The model under review builds one solid part; all positions refer to its coordinate system, in mm. Face numbers are marked on the shaded views. Coordinates: 2 decimals unless noted, no trailing zeros.
1) For P1, Ø2, axis at y = 2, z = 29.5, coming from the -X side; P2, Ø2.5, axis at x = 5, z = 64, coming from the +Y side; P3, Ø2, axis at x = -2, z = 12, coming from the +Y side; P4, Ø6, axis at x = 6, z = 89, coming from the -Y side, all flat-tipped, find the tip position at first contact; note any pin that passes through.
2) Mouldability with a two-part tool opening along X and no side actions: class the marked faces 1, 2 and 3 as released by +X, released by -X, zero draft, split by the parting line, or undercut.
3) Add section A-A, the plane z = 40.5. Give the number of separate pieces and of enclosed holes in the cut face, then the cut area to 3 significant figures.
4) For line 1 (Y direction, x = 19, z = 88); line 2 (X direction, y = -21, z = 15); line 3 (X direction, y = -11.5, z = 65), list the stretches that pass through material, from the lowest coordinate up.
from build123d import *

# Parameters (mm, degrees)
EXTRUDE_1_DEPTH = 100


with BuildPart() as part:
    # 草图1 → 凸台-拉伸1 (new body)
    with BuildSketch(Plane.XY):
        with BuildLine():
            Line((23.205623676, 19.265775848), (23.205623676, 5.365775848))
            Line((23.205623676, 5.365775848), (22.405623676, 5.365775848))
            ThreePointArc((22.405623676, 5.365775848), (22.264202319, 5.307197204), (22.205623676, 5.165775848))
            Line((22.205623676, 5.165775848), (22.205623676, 4.365775848))
            Line((22.205623676, 4.365775848), (19.005623676, 4.365775848))
            ThreePointArc((19.005623676, 4.365775848), (18.793491641, 4.453643813), (18.705623676, 4.665775848))
            Line((18.705623676, 4.665775848), (18.705623676, 6.565775848))
            ThreePointArc((18.705623676, 6.565775848), (18.793491641, 6.777907882), (19.005623676, 6.865775848))
            Line((19.005623676, 6.865775848), (20.205623676, 6.865775848))
            ThreePointArc((20.205623676, 6.865775848), (20.912730457, 7.158669066), (21.205623676, 7.865775848))
            Line((21.205623676, 7.865775848), (21.205623676, 9.515775848))
            ThreePointArc((21.205623676, 9.515775848), (20.912730457, 10.222882629), (20.205623676, 10.515775848))
            Line((20.205623676, 10.515775848), (15.137604191, 10.515775848))
            Line((15.137604191, 10.515775848), (10.905623676, 6.283795332))
            Line((10.905623676, 6.283795332), (10.905623676, -7.752243637))
            Line((10.905623676, -7.752243637), (15.137604191, -11.984224152))
            Line((15.137604191, -11.984224152), (20.205623676, -11.984224152))
            ThreePointArc((20.205623676, -11.984224152), (20.912730457, -11.691330934), (21.205623676, -10.984224152))
            Line((21.205623676, -10.984224152), (21.205623676, -9.334224152))
            ThreePointArc((21.205623676, -9.334224152), (20.912730457, -8.627117371), (20.205623676, -8.334224152))
            Line((20.205623676, -8.334224152), (19.005623676, -8.334224152))
            ThreePointArc((19.005623676, -8.334224152), (18.793491641, -8.246356187), (18.705623676, -8.034224152))
            Line((18.705623676, -8.034224152), (18.705623676, -6.134224152))
            ThreePointArc((18.705623676, -6.134224152), (18.793491641, -5.922092118), (19.005623676, -5.834224152))
            Line((19.005623676, -5.834224152), (22.205623676, -5.834224152))
            Line((22.205623676, -5.834224152), (22.205623676, -6.634224152))
            ThreePointArc((22.205623676, -6.634224152), (22.264202319, -6.775645509), (22.405623676, -6.834224152))
            Line((22.405623676, -6.834224152), (23.205623676, -6.834224152))
            Line((23.205623676, -6.834224152), (23.205623676, -20.734224152))
            ThreePointArc((23.205623676, -20.734224152), (22.473390628, -22.501991105), (20.705623676, -23.234224152))
            Line((20.705623676, -23.234224152), (6.805623676, -23.234224152))
            Line((6.805623676, -23.234224152), (6.805623676, -22.434224152))
            ThreePointArc((6.805623676, -22.434224152), (6.747045032, -22.292802796), (6.605623676, -22.234224152))
            Line((6.605623676, -22.234224152), (5.805623676, -22.234224152))
            Line((5.805623676, -22.234224152), (5.805623676, -19.034224152))
            ThreePointArc((5.805623676, -19.034224152), (5.893491641, -18.822092118), (6.105623676, -18.734224152))
            Line((6.105623676, -18.734224152), (8.005623676, -18.734224152))
            ThreePointArc((8.005623676, -18.734224152), (8.21775571, -18.822092118), (8.305623676, -19.034224152))
            Line((8.305623676, -19.034224152), (8.305623676, -20.234224152))
            ThreePointArc((8.305623676, -20.234224152), (8.598516894, -20.941330934), (9.305623676, -21.234224152))
            Line((9.305623676, -21.234224152), (10.955623676, -21.234224152))
            ThreePointArc((10.955623676, -21.234224152), (11.662730457, -20.941330934), (11.955623676, -20.234224152))
            Line((11.955623676, -20.234224152), (11.955623676, -15.166204668))
            Line((11.955623676, -15.166204668), (7.72364316, -10.934224152))
            Line((7.72364316, -10.934224152), (-6.312395809, -10.934224152))
            Line((-6.312395809, -10.934224152), (-10.544376324, -15.166204668))
            Line((-10.544376324, -15.166204668), (-10.544376324, -20.234224152))
            ThreePointArc((-10.544376324, -20.234224152), (-10.251483106, -20.941330934), (-9.544376324, -21.234224152))
            Line((-9.544376324, -21.234224152), (-7.894376324, -21.234224152))
            ThreePointArc((-7.894376324, -21.234224152), (-7.187269543, -20.941330934), (-6.894376324, -20.234224152))
            Line((-6.894376324, -20.234224152), (-6.894376324, -19.034224152))
            ThreePointArc((-6.894376324, -19.034224152), (-6.806508359, -18.822092118), (-6.594376324, -18.734224152))
            Line((-6.594376324, -18.734224152), (-4.694376324, -18.734224152))
            ThreePointArc((-4.694376324, -18.734224152), (-4.48224429, -18.822092118), (-4.394376324, -19.034224152))
            Line((-4.394376324, -19.034224152), (-4.394376324, -22.234224152))
            Line((-4.394376324, -22.234224152), (-5.194376324, -22.234224152))
            ThreePointArc((-5.194376324, -22.234224152), (-5.335797681, -22.292802796), (-5.394376324, -22.434224152))
            Line((-5.394376324, -22.434224152), (-5.394376324, -23.234224152))
            Line((-5.394376324, -23.234224152), (-19.294376324, -23.234224152))
            ThreePointArc((-19.294376324, -23.234224152), (-20.885291152, -22.66269246), (-21.748799384, -21.209416162))
            ThreePointArc((-21.748799384, -21.209416162), (-8.614181478, 8.585581001), (21.180815685, 21.720198907))
            ThreePointArc((21.180815685, 21.720198907), (22.634091983, 20.856690675), (23.205623676, 19.265775848))
        make_face()
        with BuildLine():
            Line((20.205623676, 12.265775848), (14.955623676, 12.265775848))
            ThreePointArc((14.955623676, 12.265775848), (14.071740199, 12.631892371), (13.705623676, 13.515775848))
            Line((13.705623676, 13.515775848), (13.705623676, 18.765775848))
            ThreePointArc((13.705623676, 18.765775848), (14.071740199, 19.649659324), (14.955623676, 20.015775848))
            Line((14.955623676, 20.015775848), (20.205623676, 20.015775848))
            ThreePointArc((20.205623676, 20.015775848), (21.089507152, 19.649659324), (21.455623676, 18.765775848))
            Line((21.455623676, 18.765775848), (21.455623676, 13.515775848))
            ThreePointArc((21.455623676, 13.515775848), (21.089507152, 12.631892371), (20.205623676, 12.265775848))
        make_face(mode=Mode.SUBTRACT)
        with BuildLine():
            Line((-18.794376324, -13.734224152), (-13.544376324, -13.734224152))
            ThreePointArc((-13.544376324, -13.734224152), (-12.660492848, -14.100340676), (-12.294376324, -14.984224152))
            Line((-12.294376324, -14.984224152), (-12.294376324, -20.234224152))
            ThreePointArc((-12.294376324, -20.234224152), (-12.660492848, -21.118107629), (-13.544376324, -21.484224152))
            Line((-13.544376324, -21.484224152), (-18.794376324, -21.484224152))
            ThreePointArc((-18.794376324, -21.484224152), (-19.678259801, -21.118107629), (-20.044376324, -20.234224152))
            Line((-20.044376324, -20.234224152), (-20.044376324, -14.984224152))
            ThreePointArc((-20.044376324, -14.984224152), (-19.678259801, -14.100340676), (-18.794376324, -13.734224152))
        make_face(mode=Mode.SUBTRACT)
        with BuildLine():
            Line((20.205623676, -13.734224152), (14.955623676, -13.734224152))
            ThreePointArc((14.955623676, -13.734224152), (14.071740199, -14.100340676), (13.705623676, -14.984224152))
            Line((13.705623676, -14.984224152), (13.705623676, -20.234224152))
            ThreePointArc((13.705623676, -20.234224152), (14.071740199, -21.118107629), (14.955623676, -21.484224152))
            Line((14.955623676, -21.484224152), (20.205623676, -21.484224152))
            ThreePointArc((20.205623676, -21.484224152), (21.089507152, -21.118107629), (21.455623676, -20.234224152))
            Line((21.455623676, -20.234224152), (21.455623676, -14.984224152))
            ThreePointArc((21.455623676, -14.984224152), (21.089507152, -14.100340676), (20.205623676, -13.734224152))
        make_face(mode=Mode.SUBTRACT)
        with BuildLine():
            Line((-3.738938189, -7.385981051), (-2.127784513, -4.974719175))
            ThreePointArc((-2.127784513, -4.974719175), (-2.900620909, -4.340468736), (-3.534871347, -3.567632341))
            Line((-3.534871347, -3.567632341), (-5.946133223, -5.178786017))
            ThreePointArc((-5.946133223, -5.178786017), (-6.685412585, -3.795691611), (-7.140658568, -2.294946729))
            Line((-7.140658568, -2.294946729), (-4.296381255, -1.729184795))
            ThreePointArc((-4.296381255, -1.729184795), (-4.394376324, -0.734224152), (-4.296381255, 0.26073649))
            Line((-4.296381255, 0.26073649), (-7.140658568, 0.826498424))
            ThreePointArc((-7.140658568, 0.826498424), (-6.685412585, 2.327243307), (-5.946133223, 3.710337712))
            Line((-5.946133223, 3.710337712), (-3.534871347, 2.099184036))
            ThreePointArc((-3.534871347, 2.099184036), (-2.900620909, 2.872020432), (-2.127784513, 3.50627087))
            Line((-2.127784513, 3.50627087), (-3.738938189, 5.917532746))
            ThreePointArc((-3.738938189, 5.917532746), (-2.355843783, 6.656812108), (-0.855098901, 7.112058091))
            Line((-0.855098901, 7.112058091), (-0.289336967, 4.267780778))
            ThreePointArc((-0.289336967, 4.267780778), (0.705623676, 4.365775848), (1.700584318, 4.267780778))
            Line((1.700584318, 4.267780778), (2.266346252, 7.112058091))
            ThreePointArc((2.266346252, 7.112058091), (3.767091134, 6.656812108), (5.15018554, 5.917532746))
            Line((5.15018554, 5.917532746), (3.539031864, 3.50627087))
            ThreePointArc((3.539031864, 3.50627087), (4.31186826, 2.872020432), (4.946118698, 2.099184036))
            Line((4.946118698, 2.099184036), (7.357380574, 3.710337712))
            ThreePointArc((7.357380574, 3.710337712), (8.096659936, 2.327243307), (8.551905919, 0.826498424))
            Line((8.551905919, 0.826498424), (5.707628606, 0.26073649))
            ThreePointArc((5.707628606, 0.26073649), (5.805623676, -0.734224152), (5.707628606, -1.729184795))
            Line((5.707628606, -1.729184795), (8.551905919, -2.294946729))
            ThreePointArc((8.551905919, -2.294946729), (8.096659936, -3.795691611), (7.357380574, -5.178786017))
            Line((7.357380574, -5.178786017), (4.946118698, -3.567632341))
            ThreePointArc((4.946118698, -3.567632341), (4.31186826, -4.340468736), (3.539031864, -4.974719175))
            Line((3.539031864, -4.974719175), (5.15018554, -7.385981051))
            ThreePointArc((5.15018554, -7.385981051), (3.767091134, -8.125260412), (2.266346252, -8.580506396))
            Line((2.266346252, -8.580506396), (1.700584318, -5.736229082))
            ThreePointArc((1.700584318, -5.736229082), (0.705623676, -5.834224152), (-0.289336967, -5.736229082))
            Line((-0.289336967, -5.736229082), (-0.855098901, -8.580506396))
            ThreePointArc((-0.855098901, -8.580506396), (-2.355843783, -8.125260412), (-3.738938189, -7.385981051))
        make_face(mode=Mode.SUBTRACT)
        with BuildLine():
            Line((11.955623676, 16.425008073), (11.955623676, 14.111969925))
            ThreePointArc((11.955623676, 14.111969925), (11.879503208, 13.729286493), (11.662730457, 13.404863144))
            Line((11.662730457, 13.404863144), (8.016536379, 9.758669066))
            ThreePointArc((8.016536379, 9.758669066), (7.69211303, 9.541896315), (7.309429598, 9.465775848))
            Line((7.309429598, 9.465775848), (-1.034553488, 9.465775848))
            ThreePointArc((-1.034553488, 9.465775848), (-1.95892278, 10.084276945), (-1.739845229, 11.174693022))
            ThreePointArc((-1.739845229, 11.174693022), (4.264338796, 14.811507896), (10.785263601, 17.410389951))
            ThreePointArc((10.785263601, 17.410389951), (11.599688861, 17.189978685), (11.955623676, 16.425008073))
        make_face(mode=Mode.SUBTRACT)
        with BuildLine():
            Line((-16.45360855, -11.984224152), (-14.140570402, -11.984224152))
            ThreePointArc((-14.140570402, -11.984224152), (-13.75788697, -11.908103685), (-13.433463621, -11.691330934))
            Line((-13.433463621, -11.691330934), (-9.787269543, -8.045136856))
            ThreePointArc((-9.787269543, -8.045136856), (-9.570496792, -7.720713507), (-9.494376324, -7.338030075))
            Line((-9.494376324, -7.338030075), (-9.494376324, 1.005953011))
            ThreePointArc((-9.494376324, 1.005953011), (-10.112877422, 1.930322303), (-11.203293499, 1.711244752))
            ThreePointArc((-11.203293499, 1.711244752), (-14.840108373, -4.292939273), (-17.438990428, -10.813864078))
            ThreePointArc((-17.438990428, -10.813864078), (-17.218579162, -11.628289338), (-16.45360855, -11.984224152))
        make_face(mode=Mode.SUBTRACT)
    extrude(amount=EXTRUDE_1_DEPTH)


solid = part.part
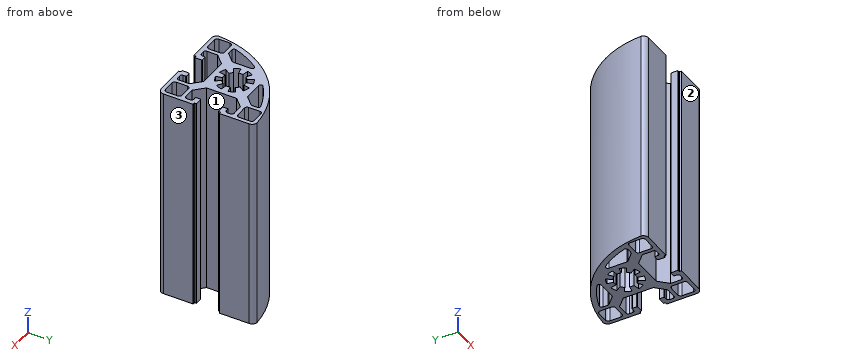
Geometry results:
1. P1: stops at x = -14.71
1. P2: stops at y = 18.45
1. P3: stops at y = 14.7
1. P4: stops at y = -23.23
2. face 1: undercut
2. face 2: zero draft
2. face 3: released by +X
3. separate pieces: 1
3. enclosed holes: 6
3. area: 691 mm2
4. line 1: y = -23.23 to -21.48, -13.73 to -11.98, -8.33 to -5.83, 4.37 to 6.87, 10.52 to 12.27, 20.02 to 21.57
4. line 2: x = -21.74 to -19.78, -12.56 to -10.19, -7.25 to -4.39, 5.81 to 8.66, 11.6 to 13.97, 21.19 to 23.19
4. line 3: x = -20.24 to -17.31, -13.24 to -6.88, 8.29 to 14.65, 21.06 to 23.21
